Check sheet for the drawn part. Datum: minimum x, y, z corner. Units: mm. A direction names the side the tool comes from. Round coordinates to 2 decimals unless told otherwise and drop trailing zeros. Write each loop counter-clockwise with the first axis right and the second up, starting at its lowest first coordinate (ties: lowest second). Pieces come first, ordered by that corner, then holes. Notation, with made-up numbers: (12.5, 24.25) - (46.5, 24.25) arc R4 ccw to (46.5, 28.25) - close; hole circle Ø5 at (19, 32.25). An arc over 180 degrees is marked (long way). Answer as a JSON object with one key per item and string values.
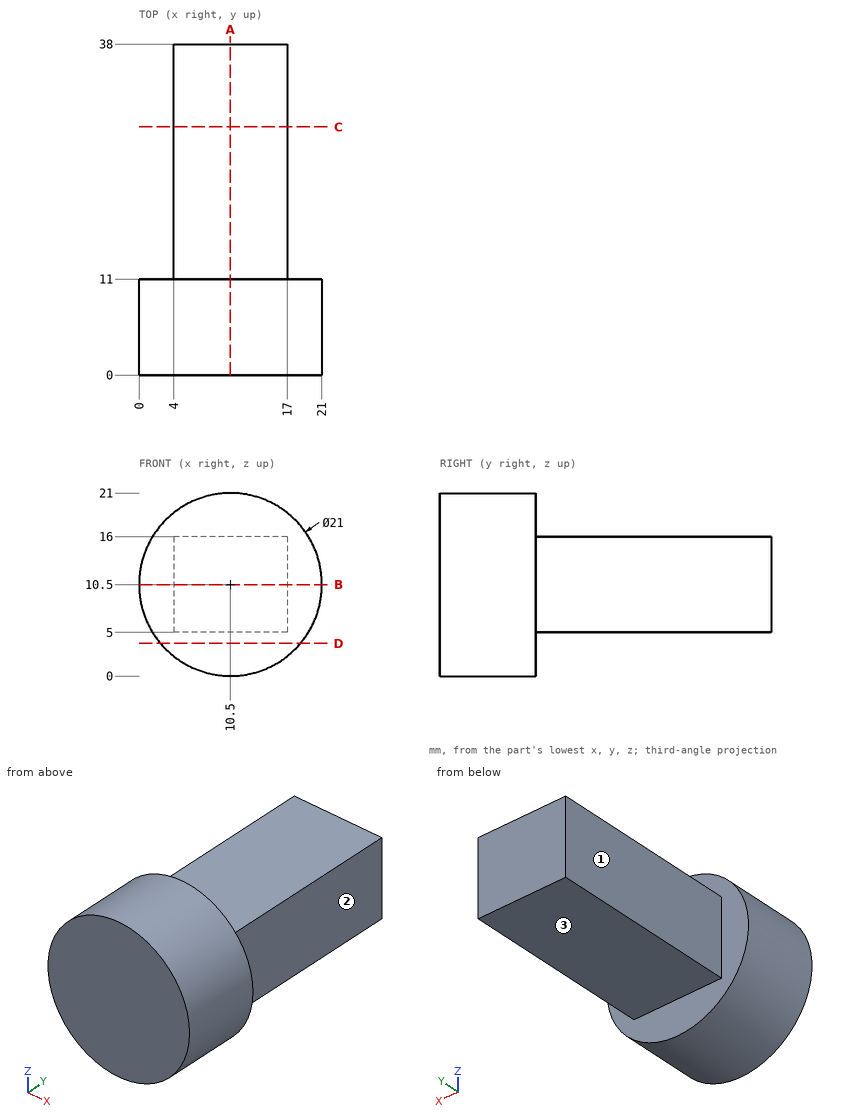
Q1. Gauge pin test, flat ends, axial feed: P1, Ø6.5, axis at x = 12.5, y = 22, coming from the -Z side; P2, Ø1, axis at y = 7.5, z = 6.5, coming from the +X side; P3, Ø2, axis at y = 14, z = 4.5, coming from the -X side. Record the tip position at first contact, or that the pin passes through.
Geometry check:
{"P1": "stops at z = 5", "P2": "stops at x = 20.4", "P3": "stops at x = 4"}
Q2. Section check D-D, the plane z = 3.75. Record the cut outline in (x, y), then the cut area to 3 significant figures.
Geometry check:
{"outline": "(2.46, 0) - (18.54, 0) - (18.54, 11) - (2.46, 11) - close", "area": "177 mm2"}
Q3. Section check A-A, the plane x = 10.5. Record the cut outline in (y, z).
Geometry check:
{"outline": "(0, 0) - (11, 0) - (11, 5) - (38, 5) - (38, 16) - (11, 16) - (11, 21) - (0, 21) - close"}
Q4. Section check C-C, the plane y = 28.5. Record the cut outline in (x, z), then the cut area to 3 significant figures.
Geometry check:
{"outline": "(4, 5) - (17, 5) - (17, 16) - (4, 16) - close", "area": "143 mm2"}
Q5. Material ranges on line 1 along Y through (x, z) = (20.25, 7.5); line 2 along X through (y, z) = (14.5, 14.75); line 3 along Z through (x, y) = (15.25, 26.5), recorded low to high. Write a range as [from, to].
Geometry check:
{"line 1": "y = [0, 11]", "line 2": "x = [4, 17]", "line 3": "z = [5, 16]"}
Q6. Set-up check for the marked faces 1, 2 and 3: record each of +Z, -Z, +X, -X, +Y, -Y from which the full face is reachable in a straight line by a thin tool's end or side.
Geometry check:
{"face 1": "+Z, -Z, -X, +Y", "face 2": "+Z, -Z, +X, +Y", "face 3": "-Z, +X, -X, +Y"}
Q7. Section check B-B, the plane z = 10.5. Record the cut outline in (x, y).
Geometry check:
{"outline": "(0, 0) - (21, 0) - (21, 11) - (17, 11) - (17, 38) - (4, 38) - (4, 11) - (0, 11) - close"}
